Could you check a few things on this model? Use its own coordinates, in mm. Round coordinates to 2 decimals unless told otherwise and drop trailing zeros. Order: outer loops, then holes, each group sorted by start corner. A loop starts at its lowest first (then second) coordinate and runs counter-clockwise, first axis right, second up. Notation, with made-up numbers: (-37, 61) - (7, 61) arc R24 cw to (7, 81) - close; hole circle Ø10 at (42, -18). An arc over 180 degrees is marked (long way). Use one line per item in the form item = value.
from build123d import *

# Parameters (mm, degrees)
BOSS_EXTRUDE1_DEPTH  = 3.175
SKETCH3_W            = 107.95
SKETCH3_H            = 3.175
CUT_EXTRUDE2_DEPTH   = 549.843544419
FILLET1_R            = 1.5875
CUT_EXTRUDE1_DEPTH   = 549.843544419
LPATTERN1_COUNT      = 3
LPATTERN1_PITCH      = 101.6
MIRROR1_COPY_1_DEPTH = 549.843544419
MIRROR1_COPY_2_DEPTH = 549.843544419
SKETCH4_R            = 1.5875
CUT_EXTRUDE3_DEPTH   = 549.843544419
LPATTERN2_COUNT      = 4
LPATTERN2_PITCH      = 76.2
SKETCH5_R            = 1.5875
SKETCH5_R_2          = 57.5
CUT_EXTRUDE4_DEPTH   = 549.843544419


with BuildPart() as part:
    # Sketch1 → Boss-Extrude1 (new body)
    with BuildSketch(Plane(origin=(0, 0, 0), x_dir=(1, 0, 0), z_dir=(0, 1, 0))):
        Polygon((401.6375, 0), (447.675, 0), (447.675, 317.5), (0, 317.5), (0, 0), (46.0375, 0), (46.0375, -3.175), (401.6375, -3.175), align=None)
    extrude(amount=BOSS_EXTRUDE1_DEPTH)

    # Sketch3 → Cut-Extrude2 (cut, through all)
    with BuildSketch(Plane(origin=(0, 3.175, 0), x_dir=(1, 0, 0), z_dir=(0, 1, 0))):
        with Locations((122.2375, 315.9125)):
            Rectangle(SKETCH3_W, SKETCH3_H)
        with Locations((325.4375, 315.9125)):
            Rectangle(SKETCH3_W, SKETCH3_H)
    extrude(amount=-CUT_EXTRUDE2_DEPTH, mode=Mode.SUBTRACT)

    # Fillet1
    fillet1_edges = [part.edges().sort_by_distance(p)[0] for p in [
        (379.4125, 1.5875, -317.5),
        (271.4625, 1.5875, -317.5),
        (176.2125, 1.5875, -317.5),
        (68.2625, 1.5875, -317.5),
        (379.4125, 1.5875, -314.325),
        (271.4625, 1.5875, -314.325),
        (176.2125, 1.5875, -314.325),
        (68.2625, 1.5875, -314.325),
        (447.675, 1.5875, -317.5),
        (447.675, 1.5875, 0),
        (0, 1.5875, 0),
        (0, 1.5875, -317.5),
        (401.6375, 1.5875, 3.175),
        (401.6375, 1.5875, 0),
        (46.0375, 1.5875, 3.175),
        (46.0375, 1.5875, 0),
    ]]
    fillet(fillet1_edges, radius=FILLET1_R - 0.0001)  # a hair under: the kernel refuses the full size

    # Sketch2 → Cut-Extrude1 (cut, through all)
    with BuildSketch(Plane(origin=(0, 3.175, 0), x_dir=(1, 0, 0), z_dir=(0, 1, 0))):
        with BuildLine():
            Line((10.795, 258.047403349), (10.795, 260.35))
            ThreePointArc((10.795, 260.35), (12.7, 262.255), (14.605, 260.35))
            Line((14.605, 260.35), (14.605, 258.047403349))
            ThreePointArc((14.605, 258.047403349), (12.7, 248.92), (10.795, 258.047403349))
        make_face()
    cut_extrude1 = extrude(amount=-CUT_EXTRUDE1_DEPTH, mode=Mode.SUBTRACT)

    # LPattern1: Cut-Extrude1 ×3
    with Locations(*[(0, 0, i * LPATTERN1_PITCH) for i in range(1, LPATTERN1_COUNT)]):
        add(cut_extrude1, mode=Mode.SUBTRACT)

    # Mirror1: Cut-Extrude1 across plane
    add(cut_extrude1.mirror(Plane.ZY.offset(-223.8375)), mode=Mode.SUBTRACT)

    # Mirror1 copy 1 sketch → Mirror1 copy 1 (cut, through all)
    with BuildSketch(Plane(origin=(447.675, 3.175, 101.6), x_dir=(-1, 0, 0), z_dir=(0, 1, 0))):
        with BuildLine():
            Line((10.795, -258.047403349), (10.795, -260.35))
            ThreePointArc((10.795, -260.35), (12.7, -262.255), (14.605, -260.35))
            Line((14.605, -260.35), (14.605, -258.047403349))
            ThreePointArc((14.605, -258.047403349), (12.7, -248.92), (10.795, -258.047403349))
        make_face()
    extrude(amount=-MIRROR1_COPY_1_DEPTH, mode=Mode.SUBTRACT)

    # Mirror1 copy 2 sketch → Mirror1 copy 2 (cut, through all)
    with BuildSketch(Plane(origin=(447.675, 3.175, 203.2), x_dir=(-1, 0, 0), z_dir=(0, 1, 0))):
        with BuildLine():
            Line((10.795, -258.047403349), (10.795, -260.35))
            ThreePointArc((10.795, -260.35), (12.7, -262.255), (14.605, -260.35))
            Line((14.605, -260.35), (14.605, -258.047403349))
            ThreePointArc((14.605, -258.047403349), (12.7, -248.92), (10.795, -258.047403349))
        make_face()
    extrude(amount=-MIRROR1_COPY_2_DEPTH, mode=Mode.SUBTRACT)

    # Sketch4 → Cut-Extrude3 (cut, through all)
    with BuildSketch(Plane(origin=(0, 3.175, 0), x_dir=(1, 0, 0), z_dir=(0, 1, 0))):
        with Locations(Location((282.575, 276.225, 0), (0, 0, 270))):
            Circle(SKETCH4_R)
        with Locations(Location((76.2, 276.225, 0), (0, 0, 270))):
            Circle(SKETCH4_R)
    cut_extrude3 = extrude(amount=-CUT_EXTRUDE3_DEPTH, mode=Mode.SUBTRACT)

    # LPattern2: Cut-Extrude3 ×4
    with Locations(*[(0, 0, i * LPATTERN2_PITCH) for i in range(1, LPATTERN2_COUNT)]):
        add(cut_extrude3, mode=Mode.SUBTRACT)

    # Sketch5 → Cut-Extrude4 (cut, through all)
    with BuildSketch(Plane(origin=(0, 3.175, 0), x_dir=(1, 0, 0), z_dir=(0, 1, 0))):
        with Locations(Location((297.65625, 276.225, 0), (0, 0, 270))):
            Circle(SKETCH5_R)
        with Locations(Location((404.01875, 276.225, 0), (0, 0, 270))):
            Circle(SKETCH5_R)
        with Locations(Location((404.01875, 169.8625, 0), (0, 0, 270))):
            Circle(SKETCH5_R)
        with Locations(Location((297.65625, 169.8625, 0), (0, 0, 270))):
            Circle(SKETCH5_R)
        with Locations(Location((350.8375, 223.04375, 0), (0, 0, 270))):
            Circle(SKETCH5_R_2)
    extrude(amount=-CUT_EXTRUDE4_DEPTH, mode=Mode.SUBTRACT)


solid = part.part
Item 1: I need wall thicknesses on L1, parallel to Z at x = 12.7, y = 1.75 (3 decimals); L2, parallel to X at y = 1.2, z = -158 (3 decimals); L3, parallel to X at y = 2.1, z = -254 (3 decimals). Which ranges of each line are inside material? Lowest first, please.
Found:
L1 = -317.5 to -262.255, -248.92 to -160.655, -147.32 to -59.055, -45.72 to 0
L2 = 0 to 10.795, 14.605 to 433.07, 436.88 to 447.675
L3 = 0 to 7.948, 17.452 to 302.382, 399.293 to 430.223, 439.727 to 447.675
Item 2: Imagine slicing it at B-B on z = -240.5. Please give me the cut outline in (x, y) (3 decimals), plus the area to 3 significant figures.
Found:
outline = (0, 0) - (296.051, 0) - (296.051, 3.175) - (0, 3.175) - close; (405.624, 0) - (447.675, 0) - (447.675, 3.175) - (405.624, 3.175) - close
area = 1,070 mm2
Item 3: Imagine slicing it at A-A on x = 342.5. Please give me the cut outline in (y, z) (3 decimals), plus the area to 3 significant figures.
Found:
outline = (0, -314.325) - (3.175, -314.325) - (3.175, -279.936) - (0, -279.936) - close; (0, -166.151) - (3.175, -166.151) - (3.175, 3.175) - (0, 3.175) - close
area = 647 mm2
Item 4: If we mould it in two halves opening along Z, with no side actions, what happens to faces 1 (the face through (434.793, 1.61, -248.923)), 2 (the face through (221, 3.175, -159)), 3 (the face through (434.793, 1.61, -147.323))? For each: released by +Z, released by -Z, zero draft, split by the parting line, or undercut.
Found:
face_1 = undercut
face_2 = zero draft
face_3 = undercut
Item 5: Imagine slicing it at C-C on y = 2.4. State how many separate pieces and enclosed holes the cut face has, plus the area to 3 significant figures.
Found:
separate_pieces = 1
enclosed_holes = 19
area = 132,000 mm2
Item 6: Will these pins go through, and if not, where does the flat tip stop? P1, Ø1.6, axis at x = 139, y = 2, coming from the -Z side (3 decimals); P2, Ø2.5, axis at x = 76.2, z = -123.825, coming from the +Y side.
Found:
P1 = -314.325
P2 = through
